```python
from build123d import *

# Parameters (mm, degrees)
SKETCH_1_R      = 3
SKETCH_1_R_2    = 2.25
EXTRUDE_1_DEPTH = 0.5
EXTRUDE_START   = -3.5
SKETCH_1_7_R    = 3
SKETCH_1_7_R_2  = 2.25
SKETCH_1_7_R_3  = 0.8
EXTRUDE_2_DEPTH = 3.5
SKETCH_1_8_R    = 2.25
SKETCH_1_8_R_2  = 0.8
SKETCH_1_8_R_3  = 0.5
EXTRUDE_3_DEPTH = 1


with BuildPart() as part:
    # Sketch 1 → Extrude 1 (new body)
    with BuildSketch(Plane(origin=(0, 0, 0), x_dir=(1, 0, 0), z_dir=(0, 1, 0))):
        with Locations(Location((0, 0, 0), (0, 0, 270))):
            Circle(SKETCH_1_R)
        with Locations(Location((0, 0, 0), (0, 0, 270))):
            Circle(SKETCH_1_R_2, mode=Mode.SUBTRACT)
    extrude(amount=EXTRUDE_1_DEPTH)

    # Sketch 1_7 → Extrude 2 (add)
    # profile 1 of 2: a face of its own
    with BuildSketch(Plane(origin=(0, 0, 0), x_dir=(1, 0, 0), z_dir=(0, 1, 0)).offset(EXTRUDE_START)):
        with Locations(Location((0, 0, 0), (0, 0, 270))):
            Circle(SKETCH_1_7_R)
        with Locations(Location((0, 0, 0), (0, 0, 270))):
            Circle(SKETCH_1_7_R_2, mode=Mode.SUBTRACT)
    # profile 2 of 2: a face of its own
    with BuildSketch(Plane(origin=(0, 0, 0), x_dir=(1, 0, 0), z_dir=(0, 1, 0)).offset(EXTRUDE_START)):
        Circle(SKETCH_1_7_R_3)
    extrude(amount=EXTRUDE_2_DEPTH)


with BuildPart() as extrude_2_kept_piece:
    # of the separate pieces the step leaves, the one the design keeps (extrude_2_pieces_kept)
    add(part.part.solids().sort_by_distance((0, 0.5, 3))[0])

    # Sketch 1_8 → Extrude 3 (add)
    # profile 1 of 2: a face of its own
    with BuildSketch(Plane(origin=(0, 0, 0), x_dir=(1, 0, 0), z_dir=(0, 1, 0))):
        with Locations(Location((0, 0, 0), (0, 0, 270))):
            Circle(SKETCH_1_8_R)
        with Locations(Location((0, 0, 0), (0, 0, 270))):
            Circle(SKETCH_1_8_R_2, mode=Mode.SUBTRACT)
    # profile 2 of 2: a face of its own
    with BuildSketch(Plane(origin=(0, 0, 0), x_dir=(1, 0, 0), z_dir=(0, 1, 0))):
        with BuildLine():
            ThreePointArc((13.5, -1.549403386), (15.049403386, 0), (13.5, 1.549403386))
            Line((13.5, 1.549403386), (2.568919841, 1.549403386))
            ThreePointArc((2.568919841, 1.549403386), (2.890221403, 0.804127004), (3, 0))
            ThreePointArc((3, 0), (2.890221403, -0.804127004), (2.568919841, -1.549403386))
            Line((2.568919841, -1.549403386), (13.5, -1.549403386))
        make_face()
        with Locations(Location((9.049403386, 0, 0), (0, 0, 270))):
            Circle(SKETCH_1_8_R_3, mode=Mode.SUBTRACT)
        with Locations(Location((11.049403386, 0, 0), (0, 0, 270))):
            Circle(SKETCH_1_8_R_3, mode=Mode.SUBTRACT)
        with Locations(Location((13.049403386, 0, 0), (0, 0, 270))):
            Circle(SKETCH_1_8_R_3, mode=Mode.SUBTRACT)
    extrude(amount=-EXTRUDE_3_DEPTH)


solid = extrude_2_kept_piece.part
```
Part model, mm, in its own coordinate system. A direction names the side the tool comes from. Round coordinates to 2 decimals unless told otherwise and drop trailing zeros. Loops run counter-clockwise (first coordinate to the right, second up) from the corner with the lowest first, then second, coordinate; pieces in that order, holes last. Notation, with made-up numbers: (41, 32.25) -> (53, 32.25) arc R20 cw to (53, 49.25) -> close; hole circle Ø9 at (-8.75, -37). An arc over 180 degrees is marked (long way). Use CSV: the item, a comma, the result in double quotes. Start each with the question number.
1) Cut at B-B, the plane z = 0.25. Give the number of separate pieces and of enclosed holes in the cut face, plus the area to 3 significant figures.
2) Cut at D-D, the plane x = 8.75. Write the cut outline in (y, z), plus the area to 3 significant figures.
3) Cut at C-C, the plane y = -2.35. Write the cut outline in (x, z), plus the area to 3 significant figures.
4) Cut at A-A, the plane x = 0. Write the cut outline in (y, z).
5) Which spindle directions (+Z, -Z, +X, -X, +Y, -Y) get a long thin tool onto all of the face, cutting with end or side? Do faces 4 (the cylindrical face through (0.676, 0.247, 2.146)), 5 (the cylindrical face through (0.676, -2.268, 2.146)), 6 (the flat face through (8, -0.5, 1.549)). Say none if no direction does.
6) Wall check: L1, parallel to X at y = -0.7, z = 0; L2, parallel to Y at x = 7, z = -0.1; L3, parallel to X at y = -1.5, z = 0. Give the ranges that are in metal, low to high. Write a range as [from, to].
7) Pull direction Z, two halves, no side cores. Call faces 1 (the flat face through (-1, -1, 0)), 2 (the flat face through (8.1, -0.5, -1.549)), 3 (the cylindrical face through (15.05, -0.49, 0.03)): +Z half, -Z half, draft (parallel to the pull), parting line (faces both ways), or undercut.
8) Drop flat-ended pins along their axis: P1, Ø1.3, axis at x = 0, z = 0, coming from the -Y side; P2, Ø2, axis at x = 0, z = 0.5, coming from the -Y side; P3, Ø0.8, axis at x = 10.5, y = -0.5, coming from the -Z side; P4, Ø1, axis at x = 9, z = 0.5, coming from the +Y side. Give the stop position or say it passes through.
Determined:
1,separate pieces,"5"
1,enclosed holes,"0"
1,area,"18.4 mm2"
2,outline,"(-1, -1.55) -> (0, -1.55) -> (0, -0.4) -> (-1, -0.4) -> close; (-1, 0.4) -> (0, 0.4) -> (0, 1.55) -> (-1, 1.55) -> close"
2,area,"2.30 mm2"
3,outline,"circle Ø6 at (0, 0); hole circle Ø4.5 at (0, 0)"
3,area,"12.4 mm2"
4,outline,"(-3.5, -3) -> (0.5, -3) -> (0.5, -2.25) -> (0, -2.25) -> (0, -0.8) -> (-1, -0.8) -> (-1, -2.25) -> (-3.5, -2.25) -> close; (-3.5, 2.25) -> (-1, 2.25) -> (-1, 0.8) -> (0, 0.8) -> (0, 2.25) -> (0.5, 2.25) -> (0.5, 3) -> (-3.5, 3) -> close"
5,face 4,"+Y"
5,face 5,"-Y"
5,face 6,"+Z, +X, +Y, -Y"
6,L1,"x = [-3, -0.8], [0.8, 8.55], [9.55, 10.55], [11.55, 12.55], [13.55, 15.05]"
6,L2,"y = [-1, 0]"
6,L3,"x = [-3, -2.25], [2.25, 3]"
7,face 1,"undercut"
7,face 2,"-Z half"
7,face 3,"parting line"
8,P1,"passes through"
8,P2,"stops at y = -1"
8,P3,"stops at z = -1.55"
8,P4,"stops at y = 0"
